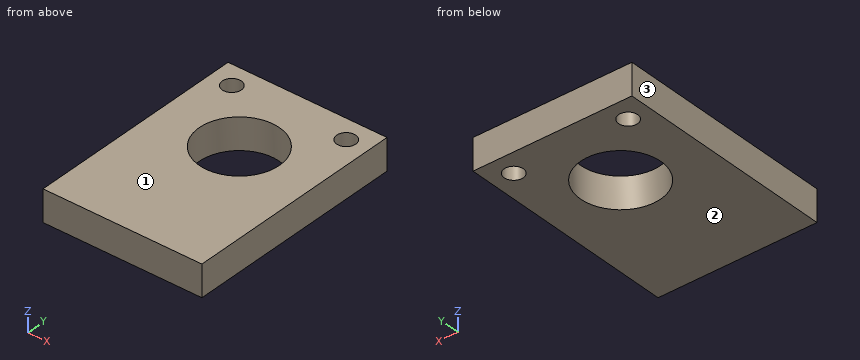
from build123d import *

# Parameters (mm, degrees)
CROQUIS1_W              = 50
CROQUIS1_H              = 70
CROQUIS1_R              = 3
SALIENTE_EXTRUIR1_DEPTH = 9.9
CROQUIS2_R              = 12.6
CORTAR_EXTRUIR1_DEPTH   = 9.9


with BuildPart() as part:
    # Croquis1 → Saliente-Extruir1 (new body)
    with BuildSketch(Plane.XY):
        Rectangle(CROQUIS1_W, CROQUIS1_H)
        with Locations(Location((-18, 28, 0), (0, 0, 180))):
            Circle(CROQUIS1_R, mode=Mode.SUBTRACT)
        with Locations(Location((18, 28, 0), (0, 0, 180))):
            Circle(CROQUIS1_R, mode=Mode.SUBTRACT)
    extrude(amount=SALIENTE_EXTRUIR1_DEPTH)

    # Croquis2 → Cortar-Extruir1 (cut)
    with BuildSketch(Plane.XY.offset(9.9)):
        with Locations((0, 9.20979846)):
            Circle(CROQUIS2_R)
    extrude(amount=-CORTAR_EXTRUIR1_DEPTH, mode=Mode.SUBTRACT)


solid = part.part
Build history of the part. All positions in model axes, mm. Face numbers are marked on the shaded views. Coordinates: 2 decimals unless noted, no trailing zeros. Write each loop counter-clockwise with the first axis right and the second up, starting at its lowest first coordinate (ties: lowest second). Pieces come first, ordered by that corner, then holes. Notation, with made-up numbers: (46.5, -8.5) -> (69.5, -8.5) arc R6 cw to (69.5, -2.5) -> close; hole circle Ø7 at (75, -31.75). An arc over 180 degrees is marked (long way). Use CSV: the item, a comma, the result in double quotes. Start each with the question number.
Q1. Drill centre lines: probe 1 along X at (y, z) = (28, 5.25); probe 2 along Y at (x, z) = (-18, 4); probe 3 along Y at (x, z) = (5, 5.25). Where is each one in solid material? Low to high.
Q2. Cut at A-A, the plane x = -18. List the corners of the cut face in (y, z).
Q3. Cut at B-B, the plane y = 28. List the corners of the cut face in (x, z), then the cut area to 3 significant figures.
Q4. Cut at C-C, the plane z = 8.75. List the corners of the cut face in (x, y).
Q5. Cut at D-D, the plane y = 2. List the corners of the cut face in (x, z).
Q6. Pull direction Z, two halves, no side cores. Call the marked faces 1, 2 and 3: released by +Z, released by -Z, zero draft, split by the parting line, or undercut.
Checked values:
1,probe 1,"x = -25 to -21, -15 to 15, 21 to 25"
1,probe 2,"y = -35 to 25, 31 to 35"
1,probe 3,"y = -35 to -2.36, 20.78 to 35"
2,outline,"(-35, 0) -> (25, 0) -> (25, 9.9) -> (-35, 9.9) -> close; (31, 0) -> (35, 0) -> (35, 9.9) -> (31, 9.9) -> close"
3,outline,"(-25, 0) -> (-21, 0) -> (-21, 9.9) -> (-25, 9.9) -> close; (-15, 0) -> (15, 0) -> (15, 9.9) -> (-15, 9.9) -> close; (21, 0) -> (25, 0) -> (25, 9.9) -> (21, 9.9) -> close"
3,area,"376 mm²"
4,outline,"(-25, -35) -> (25, -35) -> (25, 35) -> (-25, 35) -> close; hole circle Ø6 at (-18, 28); hole circle Ø25.2 at (0, 9.21); hole circle Ø6 at (18, 28)"
5,outline,"(-25, 0) -> (-10.33, 0) -> (-10.33, 9.9) -> (-25, 9.9) -> close; (10.33, 0) -> (25, 0) -> (25, 9.9) -> (10.33, 9.9) -> close"
6,face 1,"released by +Z"
6,face 2,"released by -Z"
6,face 3,"zero draft"
